Can you work these out from the model? Positions are in its coordinate system, mm. Face numbers are marked on the shaded views. A direction names the side the tool comes from. Give positions to 0.01 mm unless a question says otherwise; leave off trailing zeros. Order: outer loops, then holes, each group sorted by start corner. A loop starts at its lowest first (then second) coordinate and runs counter-clockwise, first axis right, second up. Notation, with made-up numbers: (-14, 28) - (44, 28) arc R18 cw to (44, 44) - close; hole circle Ø4 at (11, -7.5). An arc over 180 degrees is marked (long way). One line per question, with ' | ' between items.
```python
from build123d import *

# Parameters (mm, degrees)
SKETCH1_W           = 6
SKETCH1_H           = 33
BOSS_EXTRUDE1_DEPTH = 3
SKETCH3_W           = 20
SKETCH3_H           = 10
BOSS_EXTRUDE2_DEPTH = 6
FILLET1_R           = 2
CUT_EXTRUDE1_DEPTH  = 43
SKETCH5_R           = 6.05
CUT_EXTRUDE2_DEPTH  = 3.8
FILLET2_R           = 2
SKETCH6_R           = 1
CUT_EXTRUDE3_DEPTH  = 3.8
SKETCH7_R           = 1
CUT_EXTRUDE4_DEPTH  = 15
CUT_EXTRUDE5_DEPTH  = 1.7


with BuildPart() as part:
    # Sketch1 → Boss-Extrude1 (new body)
    with BuildSketch(Plane(origin=(0, 0, 0), x_dir=(1, 0, 0), z_dir=(0, 1, 0))):
        with Locations((6.921568627, 6.794117647)):
            Rectangle(SKETCH1_W, SKETCH1_H)
    extrude(amount=BOSS_EXTRUDE1_DEPTH)

    # Sketch3 → Boss-Extrude2 (add)
    with BuildSketch(Plane(origin=(9.921568627, 0, 0), x_dir=(0, 0, -1), z_dir=(1, 0, 0))):
        with Locations((6.794117647, 5)):
            Rectangle(SKETCH3_W, SKETCH3_H)
    extrude(amount=-BOSS_EXTRUDE2_DEPTH)

    # Fillet1
    fillet1_edges = [part.edges().sort_by_distance(p)[0] for p in [
        (6.921568627, 10, 3.205882353),
        (6.921568627, 10, -16.794117647),
    ]]
    fillet(fillet1_edges, radius=FILLET1_R)

    # Sketch4 → Cut-Extrude1 (cut)
    with BuildSketch(Plane.ZY.offset(-3.921568627)):
        with BuildLine():
            Line((-11.844117647, 0), (-1.744117647, 0))
            ThreePointArc((-1.744117647, 0), (-6.794117647, 5.05), (-11.844117647, 0))
        make_face()
    extrude(amount=-CUT_EXTRUDE1_DEPTH, mode=Mode.SUBTRACT)

    # Sketch5 → Cut-Extrude2 (cut)
    with BuildSketch(Plane.ZY.offset(-3.921568627)):
        with Locations((-6.794117647, 0)):
            Circle(SKETCH5_R)
    extrude(amount=-CUT_EXTRUDE2_DEPTH, mode=Mode.SUBTRACT)

    # Fillet2
    fillet2_edges = [part.edges().sort_by_distance(p)[0] for p in [
        (6.921568627, 3, -23.294117647),
        (6.921568627, 3, 9.705882353),
    ]]
    fillet(fillet2_edges, radius=FILLET2_R)

    # Sketch6 → Cut-Extrude3 (cut)
    with BuildSketch(Plane(origin=(0, 3, 0), x_dir=(1, 0, 0), z_dir=(0, 1, 0))):
        with Locations((6.921568627, -5.505882353)):
            Circle(SKETCH6_R)
        with Locations((6.921568627, 19.094117647)):
            Circle(SKETCH6_R)
    extrude(amount=-CUT_EXTRUDE3_DEPTH, mode=Mode.SUBTRACT)

    # Sketch7 → Cut-Extrude4 (cut)
    with BuildSketch(Plane(origin=(9.921568627, 0, 0), x_dir=(0, 0, -1), z_dir=(1, 0, 0))):
        with Locations((-1.705882353, 8.5)):
            Circle(SKETCH7_R)
        with Locations((15.294117647, 8.5)):
            Circle(SKETCH7_R)
    extrude(amount=-CUT_EXTRUDE4_DEPTH, mode=Mode.SUBTRACT)

    # Sketch8 → Cut-Extrude5 (cut)
    with BuildSketch(Plane.ZY.offset(-3.921568627)):
        Polygon((-0.603518724, 8.5), (0.551181815, 6.5), (2.860582891, 6.5), (4.01528343, 8.5), (2.860582891, 10.5), (0.551181815, 10.5), align=None)
        Polygon((-17.603518724, 8.5), (-16.448818185, 6.5), (-14.139417109, 6.5), (-12.98471657, 8.5), (-14.139417109, 10.5), (-16.448818185, 10.5), align=None)
    extrude(amount=-CUT_EXTRUDE5_DEPTH, mode=Mode.SUBTRACT)


solid = part.part
```
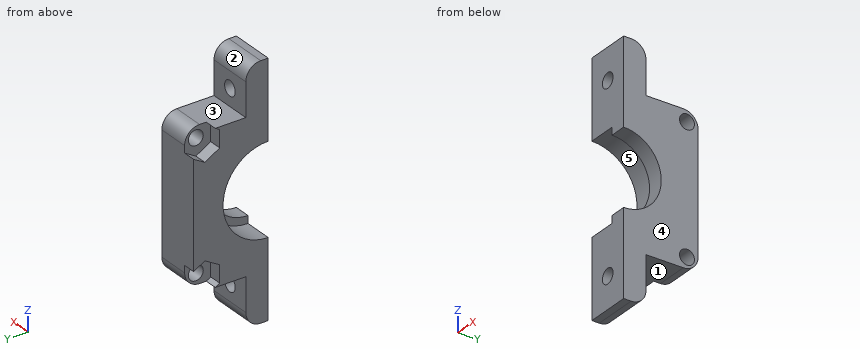
(1) Will these pins go through, and if not, where does the flat tip stop? pin 1 (1.5 mm diameter, centred on x = 6, y = 6.5, fed in from -Z); pin 2 (1.4 mm diameter, centred on x = 4.5, z = -15.5, fed in from +Y); pin 3 (2.5 mm diameter, centred on y = 8.5, z = -15.29, fed in from -X); pin 4 (5 mm diameter, centred on y = 2, z = -6, fed in from -X).
Answer below:
pin 1: z = -16.79 | pin 2: y = 6.5 | pin 3: x = 5.62 | pin 4: through
(2) Imagine slicing it at A-A (x = 7.2). List the corners of the cut face in (y, z) for me, and give its area (3 significant figures).
Answer below:
outline: (0, -23.29) - (1, -23.29) arc R2 ccw to (3, -21.29) - (3, -20.05) - (0, -20.05) - close; (0, -18.13) - (3, -18.13) - (3, -16.79) - (8, -16.79) arc R2 ccw to (10, -14.79) - (10, 1.21) arc R2 ccw to (8, 3.21) - (3, 3.21) - (3, 4.55) - (0, 4.55) - (0, -0.74) arc R6.05 cw to (0, -12.84) - close; (0, 6.47) - (3, 6.47) - (3, 7.71) arc R2 ccw to (1, 9.71) - (0, 9.71) - close; hole circle Ø2 at (8.5, -15.29); hole circle Ø2 at (8.5, 1.71) | area: 160 mm^2
(3) Imagine slicing it at C-C (y = 9). List the corners of the cut face in (x, z) for me, and give its area (3 significant figures).
Answer below:
outline: (3.92, -13.27) - (5.62, -13.27) - (5.62, -14.43) - (9.92, -14.43) - (9.92, 0.84) - (5.62, 0.84) - (5.62, -0.31) - (3.92, -0.31) - close; (5.62, -16.53) - (9.92, -16.53) - (9.92, -16.16) - (5.62, -16.16) - close; (5.62, 2.57) - (9.92, 2.57) - (9.92, 2.94) - (5.62, 2.94) - close | area: 90.8 mm^2
(4) Imagine slicing it at D-D (x = 8.8). List the corners of the cut face in (y, z) for me, and give its area (3 significant figures).
Answer below:
outline: (0, -23.29) - (1, -23.29) arc R2 ccw to (3, -21.29) - (3, -16.79) - (8, -16.79) arc R2 ccw to (10, -14.79) - (10, 1.21) arc R2 ccw to (8, 3.21) - (3, 3.21) - (3, 7.71) arc R2 ccw to (1, 9.71) - (0, 9.71) - (0, -1.74) arc R5.05 cw to (0, -11.84) - close; hole circle Ø2 at (8.5, -15.29); hole circle Ø2 at (8.5, 1.71) | area: 189 mm^2
(5) If I drill on line 1 (X direction, y = 1, z = -19); line 2 (Z direction, x = 6.55, y = 2.75); line 3 (Y direction, x = 4.4, z = 2.5), over which ranges is the centre line in solid material (lowest first)?
Answer below:
line 1: 3.92 to 5.93, 7.92 to 9.92 | line 2: -22.26 to -20.02, -18.17 to -12.18, -1.41 to 4.58, 6.43 to 8.67 | line 3: 0 to 6.5
(6) On a 3-axis mill with a long thin cutter (end or side, diameter ignored), from which of +Z, -Z, +X, -X, +Y, -Y can I reach the whole of each face in a straight line? I mean the marked faces 1 and 2. Say none if no direction works.
Answer below:
face 1: -Z, +X, -X, +Y | face 2: +Z, +X, -X, +Y
(7) If we mould it in two halves opening along Z, with no side actions, what happens to the marked faces 3, 4 and 5? For each: released by +Z, released by -Z, zero draft, split by the parting line, or undercut.
Answer below:
face 3: released by +Z | face 4: zero draft | face 5: undercut
(8) Imagine slicing it at B-B (z = -16). List the corners of the cut face in (x, y) for me, and give its area (3 significant figures).
Answer below:
outline: (3.92, 0) - (9.92, 0) - (9.92, 7.79) - (5.62, 7.79) - (5.62, 6.5) - (3.92, 6.5) - close; (5.62, 9.21) - (9.92, 9.21) - (9.92, 9.6) - (5.62, 9.6) - close | area: 46.2 mm^2
